CAD build for the part. Positions are in the model's coordinates, mm. Round coordinates to 2 decimals unless told otherwise and drop trailing zeros. Loops run counter-clockwise (first coordinate to the right, second up) from the corner with the lowest first, then second, coordinate; pieces in that order, holes last.
from build123d import *

# Parameters (mm, degrees)
SKETCH1_R           = 2.5
BOSS_EXTRUDE1_DEPTH = 45
SKETCH2_W           = 0.68
SKETCH2_H           = 0.9


with BuildPart() as part:
    # Sketch1 → Boss-Extrude1 (new body)
    with BuildSketch(Plane.XY):
        Circle(SKETCH1_R)
    extrude(amount=-BOSS_EXTRUDE1_DEPTH)

    # Sketch2 → Cut-Revolve1 (revolve, cut)
    with BuildSketch(Plane(origin=(0, 0, 0), x_dir=(0, 0, -1), z_dir=(1, 0, 0))):
        with Locations((1.91, 2.05)):
            Rectangle(SKETCH2_W, SKETCH2_H)
        with Locations((43.09, 2.05)):
            Rectangle(SKETCH2_W, SKETCH2_H)
    revolve(axis=Axis((0, 0, 0), (0, 0, -1)), mode=Mode.SUBTRACT)


solid = part.part
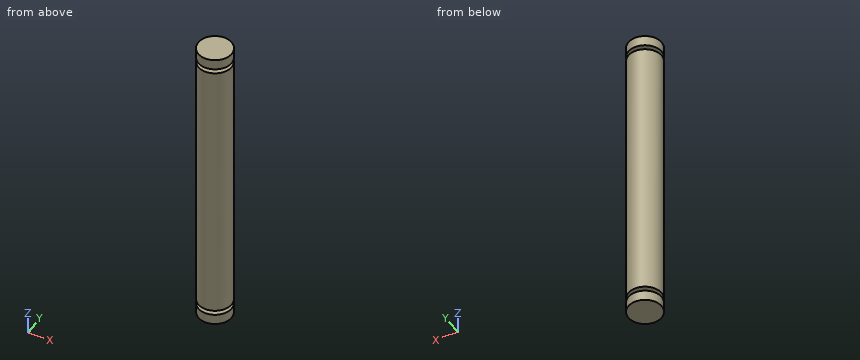
Item 1: Cut at A-A (x = -2). List the corners of the cut face in (y, z).
Verdict:
outline: (-1.5, -45) - (1.5, -45) - (1.5, -43.43) - (-1.5, -43.43) - close; (-1.5, -42.75) - (1.5, -42.75) - (1.5, -2.25) - (-1.5, -2.25) - close; (-1.5, -1.57) - (1.5, -1.57) - (1.5, 0) - (-1.5, 0) - close
Item 2: Cut at C-C (x = 0.8). List the corners of the cut face in (y, z), plus the area to 3 significant figures.
Verdict:
outline: (-2.37, -45) - (2.37, -45) - (2.37, -43.43) - (1.39, -43.43) - (1.39, -42.75) - (2.37, -42.75) - (2.37, -2.25) - (1.39, -2.25) - (1.39, -1.57) - (2.37, -1.57) - (2.37, 0) - (-2.37, 0) - (-2.37, -1.57) - (-1.39, -1.57) - (-1.39, -2.25) - (-2.37, -2.25) - (-2.37, -42.75) - (-1.39, -42.75) - (-1.39, -43.43) - (-2.37, -43.43) - close
area: 210 mm2
Item 3: Cut at B-B (z = -30.5). List the corners of the cut face in (x, y), plus the area to 3 significant figures.
Verdict:
outline: circle Ø5 at (0, 0)
area: 19.6 mm2
Item 4: Wall check: L1, parallel to Z at x = -1.8, y = 0.15; L2, parallel to Y at x = 0.15, z = -4; L3, parallel to Y at x = -1.45, z = -37.5. Give the ranges that are in metal, low to high.
Verdict:
L1: z = -45 to -43.43, -42.75 to -2.25, -1.57 to 0
L2: y = -2.5 to 2.5
L3: y = -2.04 to 2.04
Item 5: Flat gauge pins, fed straight in: P1, Ø2, axis at x = 1.5, z = -10, coming from the -Y side; P2, Ø3, axis at y = -2, z = -30.5, coming from the +X side. Where does each tip first touch, or does it go through?
Verdict:
P1: stops at y = -2.45
P2: stops at x = 2.45
